Design review of the part shown in the three views and the two pictorial views. Dimensions are in mm from the part's minimum x, y and z. Coordinates: 2 decimals unless noted, no trailing zeros. Write each loop counter-clockwise with the first axis right and the second up, starting at its lowest first coordinate (ties: lowest second). Pieces come first, ordered by that corner, then holes. Notation, with made-up numbers: (-25, 49) - (-11, 49) arc R10 cw to (-11, 56) - close; hole circle Ø3 at (49, 54). An arc over 180 degrees is marked (long way). Answer as CSV lines item,"result". Start each with the question number.
Q1. We need section D-D (y = 89). Write out the cut boundary in (x, z).
Q2. For line 1 along X through (y, z) = (61, 0.75) (1 decimal); line 2 along Y through (x, z) = (74, 1.15) (1 decimal); line 3 along Y through (x, z) = (21, 0.6) (1 decimal), list the stretches that pass through material, from the lowest coordinate up. Write a range as [from, to].
Q3. We need section A-A (y = 47.5). Write out the cut boundary in (x, z).
Q4. We need section B-B (x = 63). Write out the cut boundary in (y, z).
Q5. We need section C-C (z = 1.5). State how many separate pieces and enclosed holes the cut face has, plus the area to 3 significant figures.
Q6. Clearance check with flat-ended pins moving along their axes: pin 1 (1.2 mm diameter, centred on x = 20.3, y = 20.3, fed in from -Z); pin 2 (2.5 mm diameter, centred on x = 92, y = 50, fed in from +Z). State where each tip first meets the part, or that it passes through.
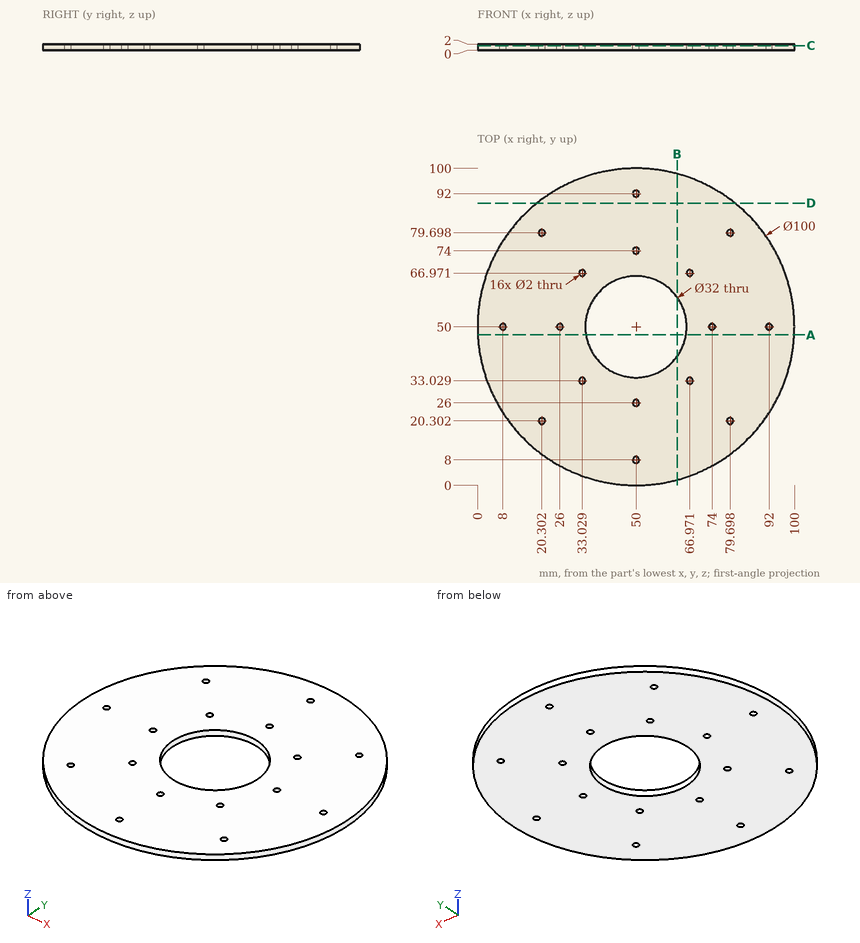
Results list:
1,outline,"(18.71, 0) - (81.29, 0) - (81.29, 2) - (18.71, 2) - close"
2,line 1,"x = [1.2, 38.4], [61.6, 98.8]"
2,line 2,"y = [6.1, 49], [51, 93.9]"
2,line 3,"y = [9.3, 19.6], [21, 79], [80.4, 90.7]"
3,outline,"(0.06, 0) - (34.2, 0) - (34.2, 2) - (0.06, 2) - close; (65.8, 0) - (99.94, 0) - (99.94, 2) - (65.8, 2) - close"
4,outline,"(1.72, 0) - (40.67, 0) - (40.67, 2) - (1.72, 2) - close; (59.33, 0) - (98.28, 0) - (98.28, 2) - (59.33, 2) - close"
5,separate pieces,"1"
5,enclosed holes,"17"
5,area,"7,000 mm2"
6,pin 1,"passes through"
6,pin 2,"stops at z = 2"
